Read the model definition and answer for the solid it produces. Units are mm, in the model's axes. A direction names the side the tool comes from. Coordinates: 2 decimals unless noted, no trailing zeros. Write each loop counter-clockwise with the first axis right and the second up, starting at its lowest first coordinate (ties: lowest second). Pieces come first, ordered by that corner, then holes. Notation, with made-up numbers: (52.5, 80.5) -> (97.5, 80.5) arc R16 ccw to (97.5, 88.5) -> close; hole circle Ø5 at (72.25, 44). An arc over 180 degrees is marked (long way). Answer in a Markdown table with one row per item. Add a question column.
Item 1: Given pin 1 Ø8 at (x, y) = (-16, -21.5) entering from +Z; pin 2 Ø10 at (x, y) = (-22.5, -17) entering from -Z; pin 3 Ø15 at (y, z) = (0, 44.45) entering from -X; pin 4 Ø4 at (y, z) = (-21.5, 28.5) entering from +X, each flat-ended and moving along its own axis, determine where each tip first touches the part or whether it passes through.
Item 2: Which of the six approach directions +Z, -Z, +X, -X, +Y, -Y give full straight-line access (tool end or side, diameter ignored) to faces 4 (the face through (39, -12, 12.7)), 5 (the face through (-25.4, 0, 32)), 6 (the face through (-12.7, -6, 52.3)), 7 (the face through (-19, -1.2, 53.9)), 8 (the face through (25.4, 0, 31))?
Item 3: Straight lines are drawn through the part: line 1 (Y direction, x = 0, z = 7.75); line 2 (Y direction, x = 16, z = 44); line 3 (X direction, y = -8, z = 66). For each, find the intervals that lie inside material, in ascending order. Write a range as from..to.
Item 4: Section B-B on x = 0 is taken. Write down the section's boundary in (y, z), then the cut area to 3 significant figures.
Item 5: For a pull along Y with two mould halves and no side action, classify faces 1 (the face through (50.507, 1.907, 6.261)), 2 (the face through (0, -25.4, 24)), 3 (the face through (-18.961, -0.559, 69.844)) as +Y half, -Y half, draft (parallel to the pull), parting line (faces both ways), or undercut.
Item 6: Section D-D on z = 63.5 is taken. Write down the section's boundary in (x, y).
Item 7: Section A-A on z = 48 is taken. Write down the section's boundary in (x, y), then the cut area to 3 significant figures.
Item 8: Section C-C on y = 0 is taken. Count the separate pieces of the cut face and the enclosed holes in it, then the cut area to 3 significant figures.
```python
from build123d import *

# Parameters (mm, degrees)
F0_R     = 63.5
F0_R_2   = 6.35
F1_DEPTH = 12.7
F3_DEPTH = 25.4
F5_DEPTH = 88.901
F4_R     = 9.525
F6_DEPTH = 88.901
F7_R     = 3.81


with BuildPart() as f1:
    # F0 (on Top) → F1 (new body)
    with BuildSketch(Plane.XY):
        Circle(F0_R)
        with Locations((0, -44.45)):
            Circle(F0_R_2, mode=Mode.SUBTRACT)
        with Locations((-44.45, 0)):
            Circle(F0_R_2, mode=Mode.SUBTRACT)
        with Locations((44.45, 0)):
            Circle(F0_R_2, mode=Mode.SUBTRACT)
        with Locations((0, 44.45)):
            Circle(F0_R_2, mode=Mode.SUBTRACT)
    extrude(amount=F1_DEPTH)

    # F2 (on Front) → F3 (join, symmetric)
    with BuildSketch(Plane.XZ):
        Polygon((-25.4, 76.2), (-25.4, 0), (25.4, 0), (25.4, 76.2), (12.7, 76.2), (12.7, 25.4), (-12.7, 25.4), (-12.7, 76.2), align=None)
    extrude(amount=F3_DEPTH, both=True)

    # F4 (on face) → F5 (cut, through all)
    with BuildSketch(Plane.YZ.offset(25.4)):
        with BuildLine():
            ThreePointArc((-25.4, 44.45), (0, 69.85), (25.4, 44.45))
            Line((25.4, 44.45), (25.4, 76.2))
            Line((25.4, 76.2), (-25.4, 76.2))
            Line((-25.4, 76.2), (-25.4, 44.45))
        make_face()
    extrude(amount=-F5_DEPTH, mode=Mode.SUBTRACT)

    # F4 (on face) → F6 (cut, through all)
    with BuildSketch(Plane.YZ.offset(25.4)):
        with Locations((0, 44.45)):
            Circle(F4_R)
    extrude(amount=-F6_DEPTH, mode=Mode.SUBTRACT)

    # F7
    f7_edges = [f1.edges().sort_by_distance(p)[0] for p in [
        (-63.5, 0, 12.7),
        (25.4, 0, 12.7),
        (0, -25.4, 12.7),
        (0, 25.4, 12.7),
        (-25.4, 0, 12.7),
    ]]
    fillet(f7_edges, radius=F7_R)


solid = f1.part
```
Results below:
| question | item | result |
|---|---|---|
| 1 | pin 1 | stops at z = 62.86 |
| 1 | pin 2 | stops at z = 0 |
| 1 | pin 3 | passes through |
| 1 | pin 4 | stops at x = 25.4 |
| 2 | face 4 | +Z |
| 2 | face 5 | +Z, -X, +Y, -Y |
| 2 | face 6 | +Z, +Y, -Y |
| 2 | face 7 | +X, -X |
| 2 | face 8 | +Z, +X, +Y, -Y |
| 3 | line 1 | y = -63.5..-50.8, -38.1..38.1, 50.8..63.5 |
| 3 | line 2 | y = -25.4..-9.51, 9.51..25.4 |
| 3 | line 3 | x = -25.4..-12.7, 12.7..25.4 |
| 4 | outline | (-63.5, 0) -> (-50.8, 0) -> (-50.8, 12.7) -> (-59.69, 12.7) arc R3.81 ccw to (-63.5, 8.89) -> close; (-38.1, 0) -> (38.1, 0) -> (38.1, 12.7) -> (29.21, 12.7) arc R3.81 cw to (25.4, 16.51) -> (25.4, 25.4) -> (-25.4, 25.4) -> (-25.4, 16.51) arc R3.81 cw to (-29.21, 12.7) -> (-38.1, 12.7) -> close; (50.8, 0) -> (63.5, 0) -> (63.5, 8.89) arc R3.81 ccw to (59.69, 12.7) -> (50.8, 12.7) -> close |
| 4 | area | 1,940 mm2 |
| 5 | face 1 | undercut |
| 5 | face 2 | -Y half |
| 5 | face 3 | parting line |
| 6 | outline | (-25.4, -16.8) -> (-12.7, -16.8) -> (-12.7, 16.8) -> (-25.4, 16.8) -> close; (12.7, -16.8) -> (25.4, -16.8) -> (25.4, 16.8) -> (12.7, 16.8) -> close |
| 7 | outline | (-25.4, -25.15) -> (-12.7, -25.15) -> (-12.7, -8.84) -> (-25.4, -8.84) -> close; (-25.4, 8.84) -> (-12.7, 8.84) -> (-12.7, 25.15) -> (-25.4, 25.15) -> close; (12.7, -25.15) -> (25.4, -25.15) -> (25.4, -8.84) -> (12.7, -8.84) -> close; (12.7, 8.84) -> (25.4, 8.84) -> (25.4, 25.15) -> (12.7, 25.15) -> close |
| 7 | area | 829 mm2 |
| 8 | separate pieces | 5 |
| 8 | enclosed holes | 0 |
| 8 | area | 2,580 mm2 |
